from build123d import *

# Parameters (mm, degrees)
BOSS_EXTRUDE2_DEPTH = 8.89
SKETCH11_R          = 19.05
CUT_EXTRUDE1_DEPTH  = 127
SKETCH12_R          = 19.05
CUT_EXTRUDE2_DEPTH  = 12.7
SKETCH13_R          = 3.175
CUT_EXTRUDE3_DEPTH  = 12.7


with BuildPart() as part:
    # Sketch1 → Boss-Extrude2 (new body)
    with BuildSketch(Plane(origin=(0, 0, 0), x_dir=(1, 0, 0), z_dir=(0, 1, 0))):
        with BuildLine():
            Line((-44.45, -50.8), (44.45, -50.8))
            ThreePointArc((44.45, -50.8), (48.940128061, -48.940128061), (50.8, -44.45))
            Line((50.8, -44.45), (50.8, 44.45))
            ThreePointArc((50.8, 44.45), (48.940128061, 48.940128061), (44.45, 50.8))
            Line((44.45, 50.8), (-44.45, 50.8))
            ThreePointArc((-44.45, 50.8), (-48.940128061, 48.940128061), (-50.8, 44.45))
            Line((-50.8, 44.45), (-50.8, -44.45))
            ThreePointArc((-50.8, -44.45), (-48.940128061, -48.940128061), (-44.45, -50.8))
        make_face()
    extrude(amount=BOSS_EXTRUDE2_DEPTH)

    # Sketch10 → Revolve1 (revolve)
    with BuildSketch(Plane.XY):
        Polygon((0, 21.59), (0, 8.89), (41.275, 8.89), (25.4, 21.59), align=None)
    revolve(axis=Axis((0, 0, 0), (0, 1, 0)))

    # Sketch11 → Cut-Extrude1 (cut)
    with BuildSketch(Plane(origin=(0, 21.59, 0), x_dir=(1, 0, 0), z_dir=(0, 1, 0))):
        with Locations((1.281459619, 50.8)):
            Circle(SKETCH11_R)
        with Locations((50.8, 0)):
            Circle(SKETCH11_R)
        with Locations((0, -50.8)):
            Circle(SKETCH11_R)
        with Locations((-50.8, 0)):
            Circle(SKETCH11_R)
    extrude(amount=-CUT_EXTRUDE1_DEPTH, mode=Mode.SUBTRACT)

    # Sketch12 → Cut-Extrude2 (cut)
    with BuildSketch(Plane(origin=(0, 21.59, 0), x_dir=(1, 0, 0), z_dir=(0, 1, 0))):
        Circle(SKETCH12_R)
    extrude(amount=-CUT_EXTRUDE2_DEPTH, mode=Mode.SUBTRACT)

    # Sketch13 → Cut-Extrude3 (cut)
    with BuildSketch(Plane(origin=(0, 8.89, 0), x_dir=(1, 0, 0), z_dir=(0, 1, 0))):
        with Locations((-38.1, 38.1)):
            Circle(SKETCH13_R)
        with Locations((38.1, 38.1)):
            Circle(SKETCH13_R)
        with Locations((38.1, -38.1)):
            Circle(SKETCH13_R)
        with Locations((-38.1, -38.1)):
            Circle(SKETCH13_R)
    extrude(amount=-CUT_EXTRUDE3_DEPTH, mode=Mode.SUBTRACT)


solid = part.part
Work out the finished part from the listing and answer in its coordinate system (mm). A direction names the side the tool comes from. Give positions to 0.01 mm unless a question says otherwise; leave off trailing zeros. Write each loop counter-clockwise with the first axis right and the second up, starting at its lowest first coordinate (ties: lowest second). Pieces come first, ordered by that corner, then holes. Notation, with made-up numbers: (-24.5, 10) - (24.5, 10) arc R14 cw to (24.5, 16) - close; hole circle Ø2 at (87, 47.5). An arc over 180 degrees is marked (long way). One line per item, written item: value. Start each with the question number.
1. Find section B-B (y = 14.75). Write down the section's boundary in (x, z), then the cut area to 3 significant figures.
2. For faces 1 (the flat face through (-37, 8.89, 32)), 2 (the flat face through (33, 4, -50.8)), 3 (the cylindrical face through (-15.12, 15.33, 11.59)), 4 (the flat face through (36, 8.89, 32)), determine the directions among +Z, -Z, +X, -X, +Y, -Y from which every point of the face is accessible in a straight line to the end or side of a thin tool.
3. Find section C-C (x = 0). Write down the section's boundary in (y, z), then the cut area to 3 significant figures.
4. Find section A-A (y = 3.75). Write down the section's boundary in (x, z) (3 decimals).
5. Given pin 1 (8.5 mm diameter, centred on x = 38.1, z = 38.1, fed in from +Y); pin 2 (5 mm diameter, centred on x = -5.5, y = 11.5, fed in from -Z); pin 3 (1.5 mm diameter, centred on y = 4.5, z = -16, fed in from -X), each flat-ended and moving along its own axis, determine where each tip first touches the part or whether it passes through.
6. Consider probe 1 along Z at (x, y) = (38.1, 5) (3 decimals); probe 2 along Z at (x, y) = (-38, 8.25); probe 3 along X at (y, z) = (3.25, -38.1) (1 decimal). Determine where each line is inside the solid, lowest interval first.
Geometry results:
1. outline: (-33.17, -7.22) arc R33.95 ccw to (-6.36, -33.35) arc R19.05 cw to (8.03, -32.99) arc R33.95 ccw to (33.17, -7.22) arc R19.05 cw to (33.17, 7.22) arc R33.95 ccw to (7.22, 33.17) arc R19.05 cw to (-7.22, 33.17) arc R33.95 ccw to (-33.17, 7.22) arc R19.05 cw to start; hole circle Ø38.1 at (0, 0)
1. area: 2,400 mm2
2. face 1: +Z, -X, +Y
2. face 2: -Z, +X, -X, +Y, -Y
2. face 3: +Y
2. face 4: +Z, +X, +Y
3. outline: (0, -31.79) - (16.48, -31.79) - (21.59, -25.4) - (21.59, -19.05) - (8.89, -19.05) - (8.89, 19.05) - (21.59, 19.05) - (21.59, 25.4) - (16.51, 31.75) - (0, 31.75) - close
3. area: 856 mm2
4. outline: (-50.8, -44.45) arc R6.35 ccw to (-44.45, -50.8) - (-17.769, -50.8) arc R19.05 cw to (20.331, -50.8) - (44.45, -50.8) arc R6.35 ccw to (50.8, -44.45) - (50.8, -19.05) arc R19.05 cw to (50.8, 19.05) - (50.8, 44.45) arc R6.35 ccw to (44.45, 50.8) - (19.05, 50.8) arc R19.05 cw to (-19.05, 50.8) - (-44.45, 50.8) arc R6.35 ccw to (-50.8, 44.45) - (-50.8, 19.05) arc R19.05 cw to (-50.8, -19.05) - close; hole circle Ø6.35 at (-38.1, -38.1); hole circle Ø6.35 at (-38.1, 38.1); hole circle Ø6.35 at (38.1, -38.1); hole circle Ø6.35 at (38.1, 38.1)
5. pin 1: y = 8.89
5. pin 2: z = -34.16
5. pin 3: x = -41.73
6. probe 1: -50.8 to -41.275, -34.925 to -14.199, 14.199 to 34.925, 41.275 to 50.8
6. probe 2: -50.8 to -41.27, -34.93 to -14.11, 14.11 to 34.93, 41.27 to 50.8
6. probe 3: -50.8 to -41.3, -34.9 to -12.9, 15.5 to 34.9, 41.3 to 50.8
